Build history of the part. All positions in model axes, mm. Give positions to 0.01 mm unless a question says otherwise; leave off trailing zeros. Write each loop counter-clockwise with the first axis right and the second up, starting at its lowest first coordinate (ties: lowest second). Pieces come first, ordered by that corner, then holes.
from build123d import *

# Parameters (mm, degrees)
EXTRUDE_1_DEPTH     = 2
SKETCH_2_R          = 2.5
CUT_EXTRUDE_1_DEPTH = 10


with BuildPart() as part:
    # 草图1 → 拉伸1 (new body)
    with BuildSketch(Plane.XY):
        with BuildLine():
            Line((0, 55), (90, 55))
            ThreePointArc((90, 55), (145, 0), (90, -55))
            Line((90, -55), (0, -55))
            ThreePointArc((0, -55), (-55, 0), (0, 55))
        make_face()
    extrude(amount=EXTRUDE_1_DEPTH)

    # 草图2 → 切除-拉伸1 (cut)
    with BuildSketch(Plane(origin=(0, 0, 0), x_dir=(-1, 0, 0), z_dir=(0, 0, -1))):
        with Locations((-90, 51)):
            Circle(SKETCH_2_R)
        with Locations((0, 51)):
            Circle(SKETCH_2_R)
        with Locations((51, 0)):
            Circle(SKETCH_2_R)
        with Locations(Location((0, -51, 0), (0, 0, 180))):
            Circle(SKETCH_2_R)
        with Locations(Location((-90, -51, 0), (0, 0, 180))):
            Circle(SKETCH_2_R)
        with Locations((-141, 0)):
            Circle(SKETCH_2_R)
    extrude(amount=-CUT_EXTRUDE_1_DEPTH, mode=Mode.SUBTRACT)


solid = part.part
1. Drill centre lines: line 1 along Y through (x, z) = (90, 1.05); line 2 along X through (y, z) = (2, 1.55); line 3 along X through (y, z) = (-1, 0.75). Where is each one in solid material? Low to high.
2. Saw through at C-C on z = 1.65. Give the cut face in (x, y), plus the area to 3 significant figures.
3. Saw through at D-D on y = -51. Give the cut face in (x, z).
4. Saw through at A-A on y = 0. Give the cut face in (x, z).
5. Saw through at B-B on x = 141. Give the cut face in (y, z).
6. Mould opens along X. For faces 1 (the face through (46, 1, 2)), 2 (the face through (-54.987, -1.209, 0.986)), 3 (the face through (92.5, 51.1, 1)) say: pulls with the +X half, pulls with the -X half, needs draft (parallel to the pull), parting line crosses it, or undercut.
7. Drop flat-ended pins along their axis: pin 1 (6.5 mm diameter, centred on x = 0, y = 51, fed in from -Z); pin 2 (1 mm diameter, centred on x = -4, z = 0.5, fed in from +Y); pin 3 (4.5 mm diameter, centred on x = 0, y = -51, fed in from +Z). Give the stop position or say it passes through.
Outcome:
1. line 1: y = -55 to -53.5, -48.5 to 48.5, 53.5 to 55
1. line 2: x = -54.96 to -52.5, -49.5 to 139.5, 142.5 to 144.96
1. line 3: x = -54.99 to -53.29, -48.71 to 138.71, 143.29 to 144.99
2. outline: (0, -55) - (90, -55) arc R55 ccw to (90, 55) - (0, 55) arc R55 ccw to start; hole circle Ø5 at (-51, 0); hole circle Ø5 at (0, -51); hole circle Ø5 at (0, 51); hole circle Ø5 at (90, -51); hole circle Ø5 at (90, 51); hole circle Ø5 at (141, 0)
2. area: 19,300 mm2
3. outline: (-20.59, 0) - (-2.5, 0) - (-2.5, 2) - (-20.59, 2) - close; (2.5, 0) - (87.5, 0) - (87.5, 2) - (2.5, 2) - close; (92.5, 0) - (110.59, 0) - (110.59, 2) - (92.5, 2) - close
4. outline: (-55, 0) - (-53.5, 0) - (-53.5, 2) - (-55, 2) - close; (-48.5, 0) - (138.5, 0) - (138.5, 2) - (-48.5, 2) - close; (143.5, 0) - (145, 0) - (145, 2) - (143.5, 2) - close
5. outline: (-20.59, 0) - (-2.5, 0) - (-2.5, 2) - (-20.59, 2) - close; (2.5, 0) - (20.59, 0) - (20.59, 2) - (2.5, 2) - close
6. face 1: needs draft
6. face 2: pulls with the -X half
6. face 3: undercut
7. pin 1: stops at z = 0
7. pin 2: stops at y = 54.89
7. pin 3: passes through
